from build123d import *

# Parameters (mm, degrees)
SKETCH1_W           = 400
SKETCH1_H           = 48
SKETCH1_R           = 2
BOSS_EXTRUDE1_DEPTH = 5
SKETCH3_W           = 42
SKETCH3_H           = 5
BOSS_EXTRUDE2_DEPTH = 100
SKETCH5_W           = 165
SKETCH5_H           = 5
BOSS_EXTRUDE3_DEPTH = 30
CUT_EXTRUDE1_DEPTH  = 408.564718787
FILLET1_R           = 10


with BuildPart() as part:
    # Sketch1 → Boss-Extrude1 (new body)
    with BuildSketch(Plane(origin=(0, 0, 0), x_dir=(1, 0, 0), z_dir=(0, 1, 0))):
        with Locations((200, -24)):
            Rectangle(SKETCH1_W, SKETCH1_H)
        with Locations(Location((20, -8, 0), (0, 0, 270))):
            Circle(SKETCH1_R, mode=Mode.SUBTRACT)
        with Locations(Location((20, -40, 0), (0, 0, 90))):
            Circle(SKETCH1_R, mode=Mode.SUBTRACT)
        with Locations(Location((292, -8, 0), (0, 0, 270))):
            Circle(SKETCH1_R, mode=Mode.SUBTRACT)
        with Locations(Location((292, -40, 0), (0, 0, 90))):
            Circle(SKETCH1_R, mode=Mode.SUBTRACT)
        with Locations(Location((52, -40, 0), (0, 0, 270))):
            Circle(SKETCH1_R, mode=Mode.SUBTRACT)
        with Locations(Location((52, -8, 0), (0, 0, 90))):
            Circle(SKETCH1_R, mode=Mode.SUBTRACT)
        with Locations(Location((260, -40, 0), (0, 0, 270))):
            Circle(SKETCH1_R, mode=Mode.SUBTRACT)
        with Locations(Location((260, -8, 0), (0, 0, 90))):
            Circle(SKETCH1_R, mode=Mode.SUBTRACT)
    extrude(amount=BOSS_EXTRUDE1_DEPTH)

    # Sketch3 → Boss-Extrude2 (add)
    with BuildSketch(Plane.ZY):
        with Locations((27, 2.5)):
            Rectangle(SKETCH3_W, SKETCH3_H)
    extrude(amount=BOSS_EXTRUDE2_DEPTH)

    # Sketch5 → Boss-Extrude3 (add)
    with BuildSketch(Plane.XY.offset(48)):
        with Locations((82.5, 2.5)):
            Rectangle(SKETCH5_W, SKETCH5_H)
    extrude(amount=BOSS_EXTRUDE3_DEPTH)

    # Sketch4 → Cut-Extrude1 (cut, through all)
    with BuildSketch(Plane(origin=(0, 5, 0), x_dir=(1, 0, 0), z_dir=(0, 1, 0))):
        with BuildLine():
            Line((-77.5, -6), (-77.5, -26))
            ThreePointArc((-77.5, -26), (-80, -28.5), (-82.5, -26))
            Line((-82.5, -26), (-82.5, -6))
            ThreePointArc((-82.5, -6), (-80, -3.5), (-77.5, -6))
        make_face()
        with BuildLine():
            Line((-17.5, -6), (-17.5, -26))
            ThreePointArc((-17.5, -26), (-20, -28.5), (-22.5, -26))
            Line((-22.5, -26), (-22.5, -6))
            ThreePointArc((-22.5, -6), (-20, -3.5), (-17.5, -6))
        make_face()
        with BuildLine():
            Line((82.5, -30), (82.5, -55))
            ThreePointArc((82.5, -55), (80, -57.5), (77.5, -55))
            Line((77.5, -55), (77.5, -30))
            ThreePointArc((77.5, -30), (80, -27.5), (82.5, -30))
        make_face()
        with BuildLine():
            Line((132.5, -30), (132.5, -55))
            ThreePointArc((132.5, -55), (130, -57.5), (127.5, -55))
            Line((127.5, -55), (127.5, -30))
            ThreePointArc((127.5, -30), (130, -27.5), (132.5, -30))
        make_face()
    extrude(amount=-CUT_EXTRUDE1_DEPTH, mode=Mode.SUBTRACT)

    # Fillet1
    fillet1_edges = [part.edges().sort_by_distance(p)[0] for p in [
        (400, 2.5, 0),
        (400, 2.5, 48),
    ]]
    fillet(fillet1_edges, radius=FILLET1_R)


solid = part.part
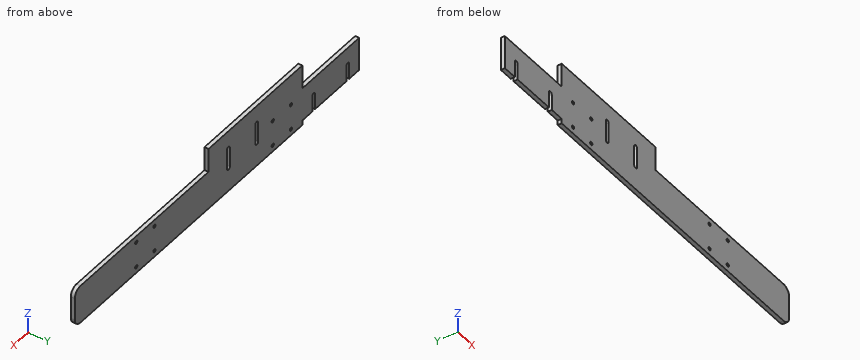
The listing builds one solid part. Answer for the finished solid, in the listing's coordinates (mm). Coordinates: 2 decimals unless noted, no trailing zeros. Loops run counter-clockwise (first coordinate to the right, second up) from the corner with the lowest first, then second, coordinate; pieces in that order, holes last. Notation, with made-up numbers: (42, 20.5) -> (48, 20.5) arc R20 ccw to (48, 41.5) -> close; hole circle Ø4 at (1.5, 78.25). An arc over 180 degrees is marked (long way). Write item = value, one per line. Start each with the question number.
1) A cutting plane is placed at B-B (y = 2.7). Count the separate pieces of the cut face and the enclosed holes in it, then the cut area to 3 significant figures.
2) A cutting plane is placed at D-D (z = 72.5). Give the vertices of the cut face in (x, y).
3) Given pin 1 Ø2.5 at (x, y) = (228.5, 3.5) entering from +Z; pin 2 Ø1.5 at (x, y) = (-53, 1.5) entering from -Z, each flat-ended and moving along its own axis, determine where each tip first touches the part or whether it passes through.
4) A cutting plane is placed at C-C (x = 306). Give the vertices of the cut face in (y, z).
5) A cutting plane is placed at A-A (z = 17). Give the vertices of the cut face in (x, y).
6) Straight lines are drawn through the part: line 1 (Z direction, x = 292, y = 2.1); line 2 (X direction, y = 0.6, z = 56.5); line 3 (Z direction, x = 298, y = 1.7). For each, find the intervals that lie inside material, in ascending order. Write a range as from..to.
Responses:
q1.separate_pieces = 1
q1.enclosed_holes = 10
q1.area = 27,700 mm²
q2.outline = (0, 0) -> (165, 0) -> (165, 5) -> (0, 5) -> close
q3.pin_1 = 48
q3.pin_2 = 6
q4.outline = (0, 0) -> (5, 0) -> (5, 48) -> (0, 48) -> close
q5.outline = (-100, 0) -> (-82.5, 0) -> (-82.5, 5) -> (-100, 5) -> close; (-77.5, 0) -> (-22.5, 0) -> (-22.5, 5) -> (-77.5, 5) -> close; (-17.5, 0) -> (400, 0) -> (400, 5) -> (-17.5, 5) -> close
q6.line_1 = 0..6, 10..38, 42..48
q6.line_2 = 0..78, 82..128, 132..165
q6.line_3 = 0..48
